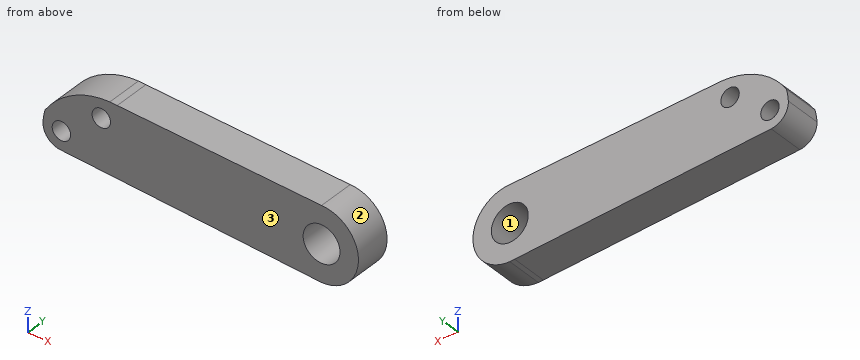
```python
from build123d import *

# Parameters (mm, degrees)
SKETCH2_R           = 1
SKETCH2_R_2         = 2
BOSS_EXTRUDE1_DEPTH = 4


with BuildPart() as part:
    # Sketch2 → Boss-Extrude1 (new body)
    with BuildSketch(Plane(origin=(0, 0, 0), x_dir=(1, 0, 0), z_dir=(0, 1, 0))):
        with BuildLine():
            ThreePointArc((-11.516754324, -1.593462652), (-8.479529409, -4.383974358), (-4.480887679, -5.395189011))
            Line((-4.480887679, -5.395189011), (-3.678548279, -5.356835657))
            Line((-3.678548279, -5.356835657), (18.483980616, -4.297424484))
            ThreePointArc((18.483980616, -4.297424484), (22.483980616, -0.297424484), (18.483980616, 3.702575516))
            Line((18.483980616, 3.702575516), (17.958963471, 3.667970452))
            Line((17.958963471, 3.667970452), (-9.863309787, 1.834141673))
            ThreePointArc((-9.863309787, 1.834141673), (-11.226928025, 1.166818548), (-11.729046011, -0.26588951))
            ThreePointArc((-11.729046011, -0.26588951), (-11.658234536, -0.935326386), (-11.516754324, -1.593462652))
        make_face()
        with Locations(Location((-5.405665929, -3.321328339, 0), (0, 0, 270))):
            Circle(SKETCH2_R, mode=Mode.SUBTRACT)
        with Locations(Location((-9.731770698, -0.161528006, 0), (0, 0, 270))):
            Circle(SKETCH2_R, mode=Mode.SUBTRACT)
        with Locations(Location((18.483980616, -0.297424484, 0), (0, 0, 270))):
            Circle(SKETCH2_R_2, mode=Mode.SUBTRACT)
    extrude(amount=BOSS_EXTRUDE1_DEPTH)


solid = part.part
```
Check sheet for the modelled part. Datum: model origin and axes. Units: mm. Face numbers are marked on the shaded views. Round coordinates to 2 decimals unless told otherwise and drop trailing zeros. Order: outer loops, then holes, each group sorted by start corner. A loop starts at its lowest first (then second) coordinate and runs counter-clockwise, first axis right, second up. Notation, with made-up numbers: (19.25, 28) -> (26.25, 28) arc R34 ccw to (26.25, 65) -> close; hole circle Ø7 at (19, 45.5). An arc over 180 degrees is marked (long way). One line per item, written item: value. Start each with the question number.
Q1. Cross-section at D-D (x = 7). Record the boundary of the cut face in (y, z).
Q2. Cross-section at A-A (z = 3.75). Record the boundary of the cut face in (x, y), and give its area (3 significant figures).
Q3. Cross-section at B-B (x = -5). Record the boundary of the cut face in (y, z), and give its area (3 significant figures).
Q4. Thickness scan on line 1 (Z direction, x = 18.5, y = 0.45); line 2 (Z direction, x = -10, y = 2.75); line 3 (X direction, y = 2.8, z = 1.5). Record the ranges inside material, lowest first.
Q5. Cross-section at C-C (y = 1.3). Record the boundary of the cut face in (x, z), and give its area (3 significant figures).
Q6. Mould release check, pull along Z, two halves, no side actions. Record for the marked faces 1, 2 and 3: pulls with the +Z half, pulls with the -Z half, needs draft (parallel to the pull), parting line crosses it, or undercut.
Q7. Gauge pin test, flat ends, axial feed: pin 1 Ø2 at (x, y) = (13, 3) entering from -Z; pin 2 Ø3 at (x, z) = (5.5, 1.5) entering from -Y; pin 3 Ø2 at (x, y) = (2, 2) entering from +Z. Record the tip position at first contact, or that the pin passes through.
Completed:
1. outline: (0, -2.95) -> (4, -2.95) -> (4, 4.85) -> (0, 4.85) -> close
2. outline: (-9.48, 0) -> (-6.31, 0) -> (-6.31, 4) -> (-9.48, 4) -> close; (-4.5, 0) -> (20.5, 0) -> (20.5, 4) -> (-4.5, 4) -> close
2. area: 113 mm²
3. outline: (0, -2.15) -> (4, -2.15) -> (4, 2.41) -> (0, 2.41) -> close; (0, 4.24) -> (4, 4.24) -> (4, 5.38) -> (0, 5.38) -> close
3. area: 22.8 mm²
4. line 1: z = -3.7 to -1.7, 2.3 to 4.3
4. line 2: z = -1.82 to -0.8, 1.12 to 3.33
4. line 3: x = -11.54 to 16.89, 20.08 to 22.3
5. outline: (-11.73, 0.27) arc R2 ccw to (-9.86, -1.83) -> (18.48, -3.7) arc R4 ccw to (18.48, 4.3) -> (-4.48, 5.4) arc R8.41 ccw to (-11.52, 1.59) arc R6.33 ccw to start; hole circle Ø2 at (-9.73, 0.16); hole circle Ø2 at (-5.41, 3.32); hole circle Ø4 at (18.48, 0.3)
5. area: 229 mm²
6. face 1: undercut
6. face 2: parting line crosses it
6. face 3: needs draft
7. pin 1: stops at z = -3.41
7. pin 2: stops at y = 0
7. pin 3: stops at z = 5.13
